from build123d import *

# Parameters (mm, degrees)
PAD002_DEPTH    = 3
SKETCH_W        = 60
SKETCH_H        = 42
PAD_DEPTH       = 9
SKETCH001_W     = 30
SKETCH001_H     = 36
PAD001_DEPTH    = 18
SKETCH002_W     = 24
SKETCH002_H     = 24
POCKET_DEPTH    = 27.001
SKETCH005_W     = 18
SKETCH005_H     = 12
POCKET001_DEPTH = 6


with BuildPart() as pad002:
    # Sketch004 → Pad002 (new body, symmetric)
    with BuildSketch(Plane.XZ):
        Polygon((9, 27), (9, 9), (30, 9), align=None)
    extrude(amount=PAD002_DEPTH, both=True)


with BuildPart() as fusion:
    # Sketch → Pad (new body)
    with BuildSketch(Plane.XY):
        Rectangle(SKETCH_W, SKETCH_H)
    extrude(amount=PAD_DEPTH)

    # Sketch001 → Pad001 (new body)
    with BuildSketch(Plane.XY.offset(9)):
        with Locations((-6, 0)):
            Rectangle(SKETCH001_W, SKETCH001_H)
    extrude(amount=PAD001_DEPTH)

    # Sketch002 → Pocket (cut, through all)
    with BuildSketch(Plane.XY.offset(27)):
        with Locations((-6, 0)):
            Rectangle(SKETCH002_W, SKETCH002_H)
    extrude(amount=-POCKET_DEPTH, mode=Mode.SUBTRACT)

    # Sketch005 → Pocket001 (cut)
    with BuildSketch(Plane.XZ.offset(18)):
        with Locations((-6, 18)):
            Rectangle(SKETCH005_W, SKETCH005_H)
    extrude(amount=-POCKET001_DEPTH, mode=Mode.SUBTRACT)

    # Fusion: union Pad002
    add(pad002.part)


solid = fusion.part
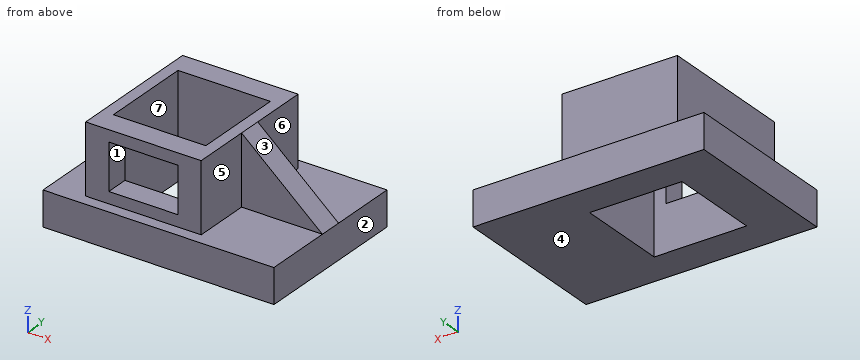
Here's how the part is built. I have some questions about the finished solid (model axes, mm). Face numbers are marked on the shaded views. A direction names the side the tool comes from. Coordinates: 2 decimals unless noted, no trailing zeros. Order: outer loops, then holes, each group sorted by start corner. A loop starts at its lowest first (then second) coordinate and runs counter-clockwise, first axis right, second up. Notation, with made-up numbers: (58, 26) - (65, 26) arc R9 cw to (65, 33) - close; hole circle Ø3 at (81, 80.25). An arc over 180 degrees is marked (long way). Use CSV: the item, a comma, the result in double quotes. Start each with the question number.
1. I'm going to push flat-ended pins straight in: pin 1 (14.5 mm diameter, centred on y = 4.5, z = 19.5, fed in from -X); pin 2 (6 mm diameter, centred on x = 17, z = 22.5, fed in from -Y); pin 3 (1.5 mm diameter, centred on x = 1, z = 15.5, fed in from +Y). Where does each tip first touch, or does it pass through?
2. For the marked faces 5, 6 and 7, which set-ups out of +Z, -Z, +X, -X, +Y, -Y let a thin tool reach every point of the face, with its end or its side?
3. Suppose I cut it at C-C on x = -13. List the corners of the cut face in (y, z) for me, then the cut area to 3 significant figures.
4. If we mould it in two halves opening along Z, with no side actions, what happens to the marked faces 1, 2, 3 and 4? For each: +Z half, -Z half, draft (parallel to the pull), parting line (faces both ways), or undercut.
5. Suppose I cut it at A-A on y = -2. List the corners of the cut face in (x, z) for me, then the cut area to 3 significant figures.
6. Suppose I cut it at D-D on y = 13.5. List the corners of the cut face in (x, z) for me, then the cut area to 3 significant figures.
7. Suppose I cut it at B-B on z = 25.5. List the corners of the cut face in (x, y) for me.
8. Please list where these lines run through material, in increasing order: line 1 (Z direction, x = -6, y = -13); line 2 (X direction, y = -2.5, z = 1.25); line 3 (X direction, y = -12.5, z = 22.5). Write a range as from..to.
Output:
1,pin 1,"stops at x = -21"
1,pin 2,"stops at y = -3"
1,pin 3,"stops at y = 18"
2,face 5,"+Z, +X, -Y"
2,face 6,"+Z, +X, +Y"
2,face 7,"+Z, -Z"
3,outline,"(-21, 0) - (-12, 0) - (-12, 12) - (-18, 12) - (-18, 9) - (-21, 9) - close; (-18, 24) - (-12, 24) - (-12, 27) - (-18, 27) - close; (12, 0) - (21, 0) - (21, 9) - (18, 9) - (18, 27) - (12, 27) - close"
3,area,"306 mm2"
4,face 1,"undercut"
4,face 2,"draft"
4,face 3,"+Z half"
4,face 4,"-Z half"
5,outline,"(-30, 0) - (-18, 0) - (-18, 27) - (-21, 27) - (-21, 9) - (-30, 9) - close; (6, 0) - (30, 0) - (30, 9) - (9, 27) - (6, 27) - close"
5,area,"621 mm2"
6,outline,"(-30, 0) - (30, 0) - (30, 9) - (9, 9) - (9, 27) - (-21, 27) - (-21, 9) - (-30, 9) - close"
6,area,"1,080 mm2"
7,outline,"(-21, -18) - (9, -18) - (9, -3) - (10.75, -3) - (10.75, 3) - (9, 3) - (9, 18) - (-21, 18) - close; hole (-18, -12) - (6, -12) - (6, 12) - (-18, 12) - close"
8,line 1,"z = 0..12, 24..27"
8,line 2,"x = -30..-18, 6..30"
8,line 3,"x = -21..-15, 3..9"
